Read the model definition and answer for the solid it produces. Units are mm, in the model's axes. Face numbers are marked on the shaded views. A direction names the side the tool comes from. Coordinates: 2 decimals unless noted, no trailing zeros. Loops run counter-clockwise (first coordinate to the right, second up) from the corner with the lowest first, then second, coordinate; pieces in that order, holes last.
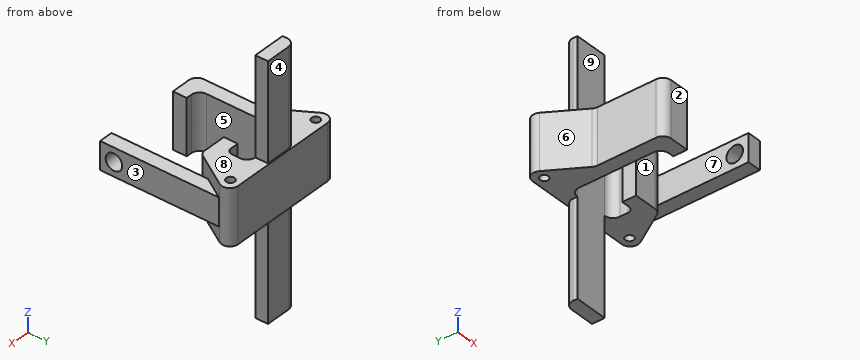
from build123d import *

# Parameters (mm, degrees)
EXTRUDE_THIN1_DEPTH = 20
BOSS_EXTRUDE1_DEPTH = 20
FILLET1_R           = 3
CUT_EXTRUDE1_REACH  = 55.346
SKETCH4_R           = 1.5
FILLET2_R           = 3
FILLET3_R           = 2
SKETCH5_W           = 12
SKETCH5_H           = 4.580516002
BOSS_EXTRUDE2_DEPTH = 35
BOSS_EXTRUDE3_START = -55
SKETCH5_2_W         = 12
SKETCH5_2_H         = 4.580516002
BOSS_EXTRUDE3_DEPTH = 35
FILLET4_R           = 3
BOSS_EXTRUDE4_START = -5
SKETCH6_W           = 5
SKETCH6_H           = 43
BOSS_EXTRUDE4_DEPTH = 10
SKETCH7_R           = 3
CUT_EXTRUDE2_DEPTH  = 5


with BuildPart() as part:
    # Sketch2 → Extrude-Thin1 (new body)
    with BuildSketch(Plane.XY):
        Polygon((-13, -33), (-18, -33), (-18, 0), (0, 0), (0, -8), (-5, -8), (-5, -13), (5, -13), (5, 5), (-23, 5), (-23, -38), (-13, -38), align=None)
    extrude(amount=EXTRUDE_THIN1_DEPTH)

    # Sketch3 → Boss-Extrude1 (add)
    with BuildSketch(Plane.XY.offset(20)):
        Polygon((5, 5), (16, 5), (5, -13), align=None)
        Polygon((-23, 5), (-34, 5), (-23, -13), align=None)
    extrude(amount=-BOSS_EXTRUDE1_DEPTH)

    # Fillet1
    fillet1_edges = [part.edges().sort_by_distance(p)[0] for p in [
        (-23, -38, 10),
        (5, -13, 10),
        (-18, -33, 10),
        (16, 5, 10),
        (-34, 5, 10),
        (-23, -13, 10),
    ]]
    fillet(fillet1_edges, radius=FILLET1_R)

    # Sketch4 → Cut-Extrude1 (cut, up to next)
    with BuildSketch(Plane.XY.offset(20), mode=Mode.PRIVATE) as cut_extrude1_sk1:
        with Locations((9.759301062, 1.5)):
            Circle(SKETCH4_R)
    cut_extrude1_tool1 = extrude(cut_extrude1_sk1.sketch, amount=-CUT_EXTRUDE1_REACH, mode=Mode.PRIVATE) & part.part
    # Sketch4 → Cut-Extrude1 (cut, up to next)
    with BuildSketch(Plane.XY.offset(20), mode=Mode.PRIVATE) as cut_extrude1_sk2:
        with Locations((-27.759301062, 1.5)):
            Circle(SKETCH4_R)
    cut_extrude1_tool2 = extrude(cut_extrude1_sk2.sketch, amount=-CUT_EXTRUDE1_REACH, mode=Mode.PRIVATE) & part.part
    add(cut_extrude1_tool1.solids().sort_by_distance((9.759301, 1.5, 20))[0], mode=Mode.SUBTRACT)
    add(cut_extrude1_tool2.solids().sort_by_distance((-27.759301, 1.5, 20))[0], mode=Mode.SUBTRACT)

    # Fillet2
    fillet2_edges = [part.edges().sort_by_distance(p)[0] for p in [
        (0, 0, 10),
        (-18, 0, 10),
    ]]
    fillet(fillet2_edges, radius=FILLET2_R)

    # Fillet3
    fillet3_edges = [part.edges().sort_by_distance(p)[0] for p in [
        (0, -8, 10),
    ]]
    fillet(fillet3_edges, radius=FILLET3_R)

    # Sketch5 → Boss-Extrude2 (add)
    with BuildSketch(Plane.XY.offset(20)):
        with Locations((-9, 2.290258001)):
            Rectangle(SKETCH5_W, SKETCH5_H)
    extrude(amount=BOSS_EXTRUDE2_DEPTH)

    # Sketch5<2> → Boss-Extrude3 (add)
    with BuildSketch(Plane.XY.offset(20).offset(BOSS_EXTRUDE3_START)):
        with Locations((-9, 2.290258001)):
            Rectangle(SKETCH5_2_W, SKETCH5_2_H)
    extrude(amount=BOSS_EXTRUDE3_DEPTH)

    # Fillet4
    fillet4_edges = [part.edges().sort_by_distance(p)[0] for p in [
        (-15, 4.580516002, 37.5),
        (-15, 4.580516002, -17.5),
    ]]
    fillet(fillet4_edges, radius=FILLET4_R)

    # Sketch6 → Boss-Extrude4 (add)
    with BuildSketch(Plane.XY.offset(20).offset(BOSS_EXTRUDE4_START)):
        with Locations((10.444444444, -21.5)):
            Rectangle(SKETCH6_W, SKETCH6_H)
    extrude(amount=-BOSS_EXTRUDE4_DEPTH)

    # Sketch7 → Cut-Extrude2 (cut)
    with BuildSketch(Plane(origin=(12.944444444, 0, 0), x_dir=(0, 0, -1), z_dir=(1, 0, 0))):
        with Locations(Location((-10, -38, 0), (0, 0, 90))):
            Circle(SKETCH7_R)
    extrude(amount=-CUT_EXTRUDE2_DEPTH, mode=Mode.SUBTRACT)


solid = part.part
Item 1: A cutting plane is placed at D-D on x = -1. Determine the outline of the cut face in (y, z).
Numbers:
outline: (-13, 0) - (-7.73, 0) - (-7.73, 20) - (-13, 20) - close; (-0.76, 0) - (5, 0) - (5, 20) - (-0.76, 20) - close
Item 2: A cutting plane is placed at B-B on z = 10. Give the number of separate pieces and of enclosed holes in the cut face, then the cut area to 3 significant figures.
Numbers:
separate pieces: 2
enclosed holes: 2
area: 785 mm2
Item 3: A cutting plane is placed at A-A on y = -20. Determine the outline of the cut face in (x, z), then the cut area to 3 significant figures.
Numbers:
outline: (-23, 0) - (-18, 0) - (-18, 20) - (-23, 20) - close; (7.94, 5) - (12.94, 5) - (12.94, 15) - (7.94, 15) - close
area: 150 mm2
Item 4: Find the intervals of material crossed by line 1 along Y through (x, z) = (-15, 14.5); line 2 along X through (y, z) = (-23, 10.5); line 3 along Z through (x, y) = (-19, 1), in increasing order.
Numbers:
line 1: y = -38 to -33, 0 to 5
line 2: x = -23 to -18, 7.94 to 12.94
line 3: z = 0 to 20
Item 5: Which of the six approach directions +Z, -Z, +X, -X, +Y, -Y give full straight-line access (tool end or side, diameter ignored) to the marked faces 1, 2, 3, 4 and 5?
Numbers:
face 1: +Z, -Z, -Y
face 2: +Z, -Z, -X, -Y
face 3: +Z, -Z, +X, -Y
face 4: +Z, +X, -X, +Y
face 5: +Z, -Z
Item 6: Given pin 1 (12 mm diameter, centred on x = -10, z = 42.5, fed in from -Y); pin 2 (1.5 mm diameter, centred on y = -34.5, z = 12.5, fed in from +X); pin 3 (1.3 mm diameter, centred on y = 1, z = 31, fed in from -X), each flat-ended and moving along its own axis, determine where each tip first touches the part or whether it passes through.
Numbers:
pin 1: stops at y = 0
pin 2: stops at x = 12.94
pin 3: stops at x = -15
Item 7: A cutting plane is placed at C-C on y = -37. Determine the outline of the cut face in (x, z), then the cut area to 3 significant figures.
Numbers:
outline: (-22.24, 0) - (-13, 0) - (-13, 20) - (-22.24, 20) - close; (7.94, 5) - (12.94, 5) - (12.94, 7.17) - (7.94, 7.17) - close; (7.94, 12.83) - (12.94, 12.83) - (12.94, 15) - (7.94, 15) - close
area: 206 mm2
Item 8: Determine the mould class of the marked faces 6, 7, 8 and 9 for opening direction X: released by +X, released by -X, zero draft, split by the parting line, or undercut.
Numbers:
face 6: released by -X
face 7: undercut
face 8: zero draft
face 9: undercut
